Geometry check sheet. Reference: drawing and pictorial views, mm from the part's lowest x, y, z. A direction names the side the tool comes from. Give positions to 0.01 mm unless a question says otherwise; leave off trailing zeros. Write each loop counter-clockwise with the first axis right and the second up, starting at its lowest first coordinate (ties: lowest second). Pieces come first, ordered by that corner, then holes.
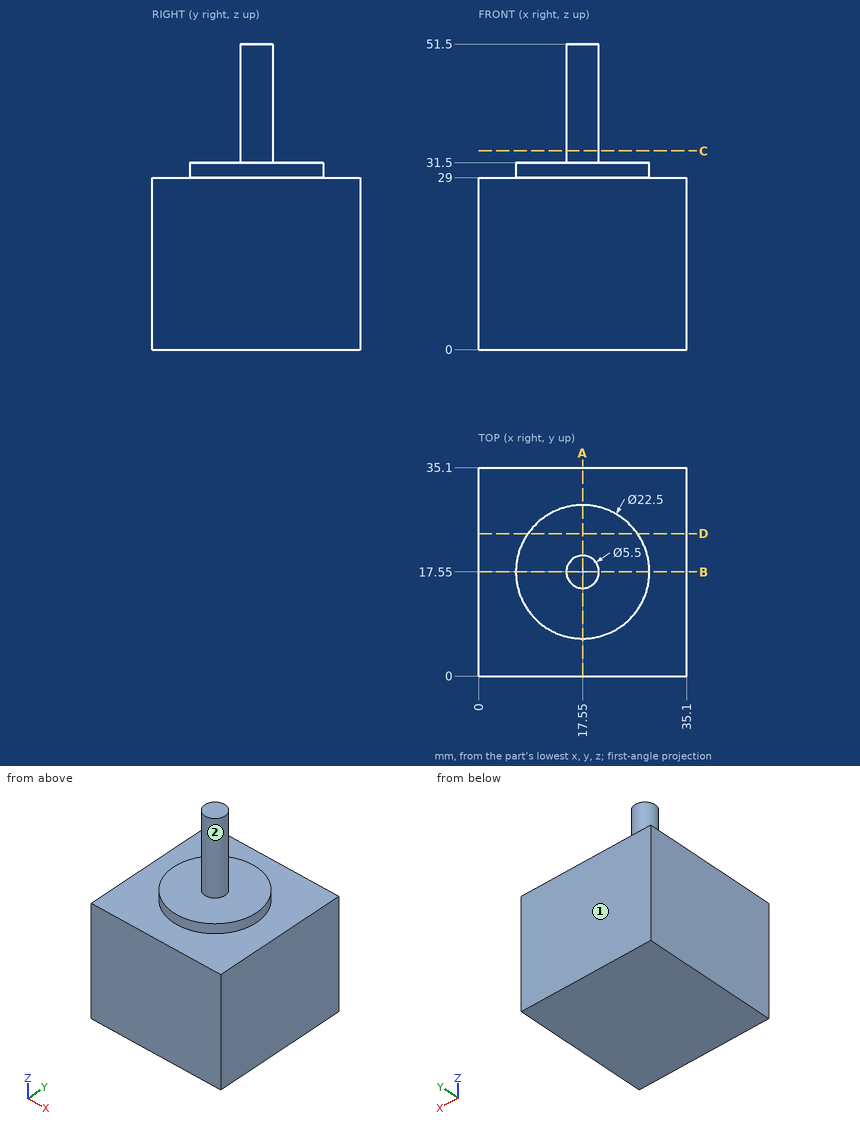
Item 1: Depth check by flat-ended pin: pin 1 (10 mm diameter, centred on x = 25, z = 45.5, fed in from -Y); pin 2 (1 mm diameter, centred on y = 20, z = 46, fed in from +X); pin 3 (3 mm diameter, centred on y = 25, z = 31, fed in from +X). Enter the tip coordinate at first touch or a pass-through.
Answer key:
pin 1: stops at y = 16.3
pin 2: stops at x = 19.49
pin 3: stops at x = 27.1
Item 2: Sectioned sample at A-A on x = 17.55. Record the cut outline in (y, z), then the cut area to 3 significant figures.
Answer key:
outline: (0, 0) - (35.1, 0) - (35.1, 29) - (28.8, 29) - (28.8, 31.5) - (20.3, 31.5) - (20.3, 51.5) - (14.8, 51.5) - (14.8, 31.5) - (6.3, 31.5) - (6.3, 29) - (0, 29) - close
area: 1,180 mm2
Item 3: Set-up check for the marked faces 1 and 2: record each of +Z, -Z, +X, -X, +Y, -Y from which the full face is reachable in a straight line by a thin tool's end or side.
Answer key:
face 1: +Z, -Z, +X, -X, +Y
face 2: +Z
Item 4: Sectioned sample at D-D on y = 24. Record the cut outline in (x, z).
Answer key:
outline: (0, 0) - (35.1, 0) - (35.1, 29) - (26.77, 29) - (26.77, 31.5) - (8.33, 31.5) - (8.33, 29) - (0, 29) - close
Item 5: Sectioned sample at C-C on z = 33.5. Record the cut outline in (x, y).
Answer key:
outline: circle Ø5.5 at (17.55, 17.55)
Item 6: Scan lines: line 1 along Z through (x, y) = (6, 32); line 2 along Z through (x, y) = (12, 14); line 3 along X through (y, z) = (15.5, 42). Record each from-to range of solid material in increasing order.
Answer key:
line 1: z = 0 to 29
line 2: z = 0 to 31.5
line 3: x = 15.72 to 19.38
